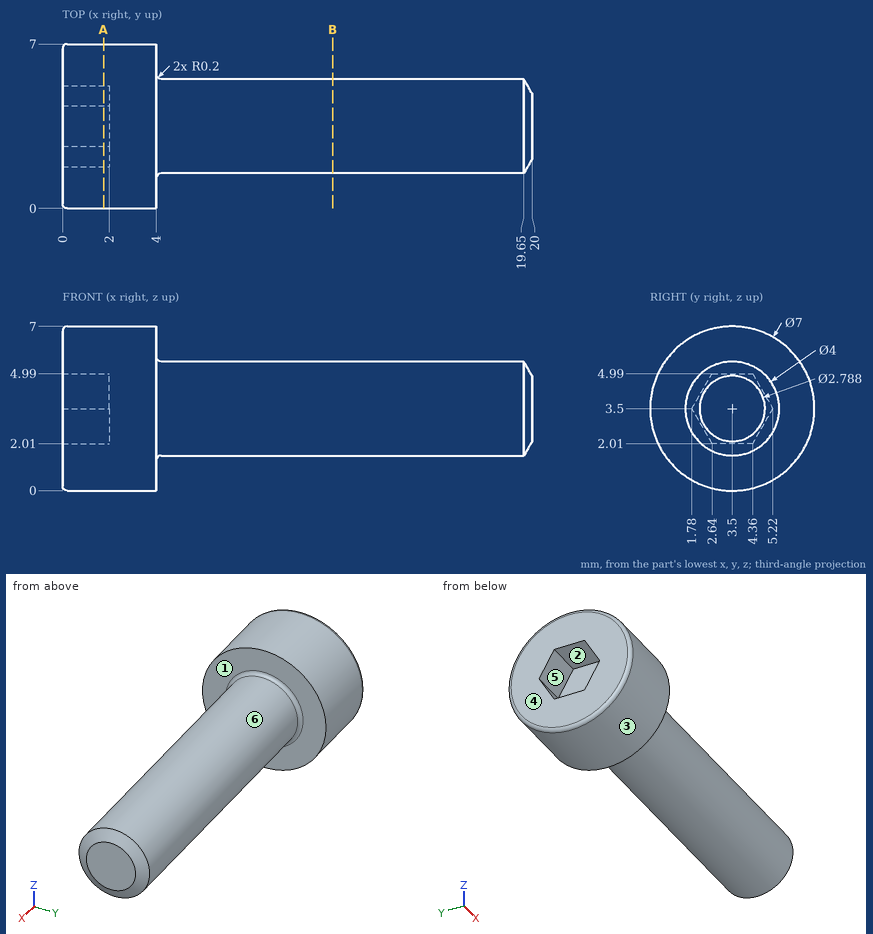
Check sheet for the drawn part. Datum: minimum x, y, z corner. Units: mm. A direction names the side the tool comes from. Round coordinates to 2 decimals unless told otherwise and drop trailing zeros. Order: outer loops, then holes, each group sorted by start corner. A loop starts at its lowest first (then second) coordinate and runs counter-clockwise, first axis right, second up.
(1) Scan lines: probe 1 along X at (y, z) = (3, 2.5); probe 2 along Y at (x, z) = (13.5, 3.5); probe 3 along X at (y, z) = (1.25, 4.5). Record each from-to range of solid material in increasing order.
(2) Draft check along Y on the marked faces 4, 5 and 6. Enter one of: pulls with the +Y half, pulls with the -Y half, needs draft (parallel to the pull), parting line crosses it, or undercut.
(3) Go/stop test with flat-tipped pins: P1, Ø3, axis at x = 17.5, y = 1.5, coming from the -Z side; P2, Ø0.9, axis at y = 3.5, z = 4, coming from the -X side; P3, Ø1.5, axis at x = 3, y = 1.5, coming from the +Z side; P4, Ø0.9, axis at x = 1, y = 4, coming from the +Z side. Record where each tip stops, or that it passes through.
(4) Access from +Z, -Z, +X, -X, +Y, -Y to the whole of each face (thin tool, end or side, straight path). Record for the marked faces 1, 2 and 3.
(5) Cross-section at B-B, the plane x = 11.5. Enter the section's corners in (y, z).
(6) Cross-section at A-A, the plane x = 1.75. Enter the section's corners in (y, z), and give its area (3 significant figures).
Check sheet entries:
1. probe 1: x = 2 to 20
1. probe 2: y = 1.5 to 5.5
1. probe 3: x = 0 to 4
2. face 4: needs draft
2. face 5: undercut
2. face 6: parting line crosses it
3. P1: stops at z = 1.56
3. P2: stops at x = 2
3. P3: stops at z = 6.77
3. P4: stops at z = 7
4. face 1: +X
4. face 2: -X
4. face 3: +X, -X
5. outline: circle Ø4 at (3.5, 3.5)
6. outline: circle Ø7 at (3.5, 3.5); hole (1.78, 3.5) - (2.64, 2.01) - (4.36, 2.01) - (5.22, 3.5) - (4.36, 4.99) - (2.64, 4.99) - close
6. area: 30.8 mm2
